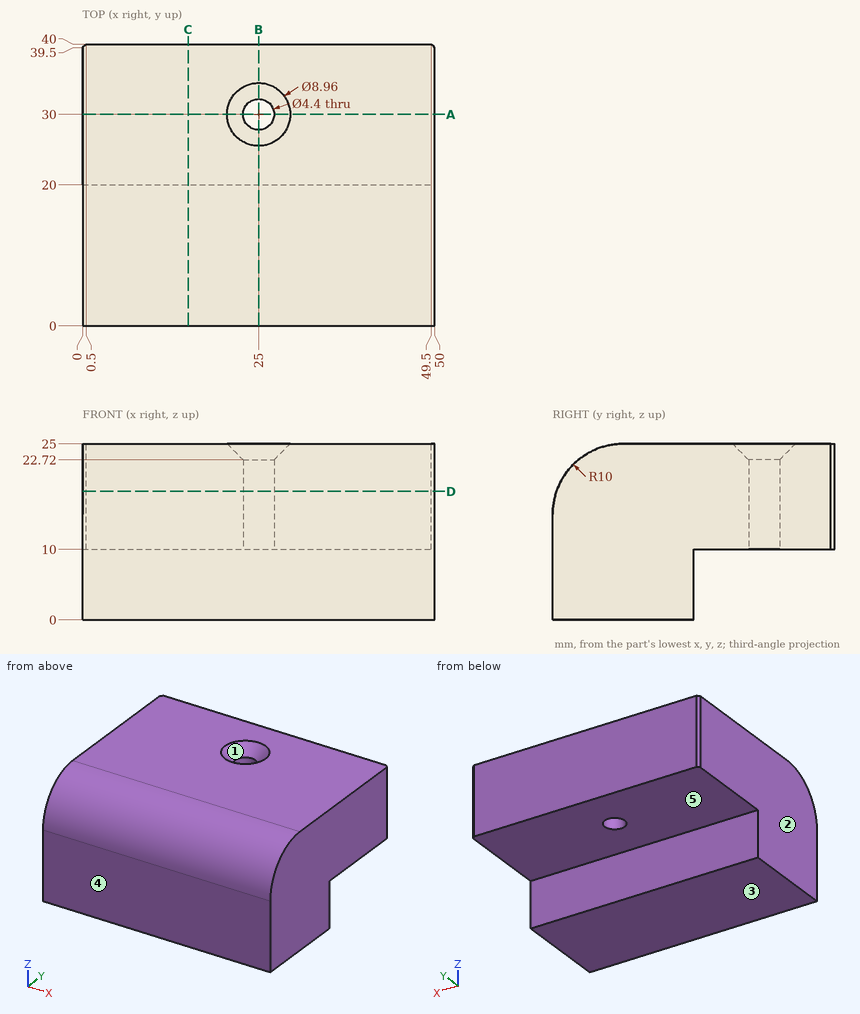
Study the drawing (mm; zero at the part's minimum x, y, z) and answer. A direction names the side the tool comes from. Coordinates: 2 decimals unless noted, no trailing zeros. Write each loop counter-clockwise with the first axis right and the second up, starting at its lowest first coordinate (ties: lowest second). Pieces come first, ordered by that corner, then holes. Notation, with made-up numbers: (-22.5, 50) - (-12.5, 50) arc R36 cw to (-12.5, 85) - close; hole circle Ø11 at (-6.75, 7). An arc over 180 degrees is marked (long way). Put each result on its own line as item: value.
1. Determine the mould class of the marked faces 1, 2 and 3 for opening direction X: pulls with the +X half, pulls with the -X half, needs draft (parallel to the pull), parting line crosses it, or undercut.
Answer sheet:
face 1: undercut
face 2: pulls with the -X half
face 3: needs draft
2. The part is cut by section C-C on x = 15. Give the vertices of the cut face in (y, z).
Answer sheet:
outline: (0, 0) - (20, 0) - (20, 10) - (40, 10) - (40, 25) - (10, 25) arc R10 ccw to (0, 15) - close
3. Find the intervals of material crossed by line 1 along Y through (x, z) = (25, 15); line 2 along X through (y, z) = (30, 16); line 3 along Z through (x, y) = (42, 29), in increasing order. Write a range as from..to.
Answer sheet:
line 1: y = 0..27.8, 32.2..40
line 2: x = 0..22.8, 27.2..50
line 3: z = 10..25
4. The part is cut by section B-B on x = 25. Give the vertices of the cut face in (y, z).
Answer sheet:
outline: (0, 0) - (20, 0) - (20, 10) - (27.8, 10) - (27.8, 22.72) - (25.52, 25) - (10, 25) arc R10 ccw to (0, 15) - close; (32.2, 10) - (40, 10) - (40, 25) - (34.48, 25) - (32.2, 22.72) - close
5. The part is cut by section A-A on y = 30. Give the vertices of the cut face in (x, z).
Answer sheet:
outline: (0, 10) - (22.8, 10) - (22.8, 22.72) - (20.52, 25) - (0, 25) - close; (27.2, 10) - (50, 10) - (50, 25) - (29.48, 25) - (27.2, 22.72) - close
6. A tool of negligible diameter and unlimited length cuts with its end or side. For the marked faces 4 and 5, from which of +Z, -Z, +X, -X, +Y, -Y can it reach the whole face along a straight path? Write none if from no direction.
Answer sheet:
face 4: +Z, -Z, +X, -X, -Y
face 5: -Z, +X, -X, +Y
7. The part is cut by section D-D on z = 18.25. Give the vertices of the cut face in (x, y), plus the area to 3 significant figures.
Answer sheet:
outline: (0, 0.54) - (50, 0.54) - (50, 39.5) - (49.5, 40) - (0.5, 40) - (0, 39.5) - close; hole circle Ø4.4 at (25, 30)
area: 1,960 mm^2
8. Flat-ended cylindrical pins translate along their axes: pin 1 Ø5 at (x, y) = (25, 30) entering from -Z; pin 2 Ø8 at (y, z) = (30.5, 4.5) entering from -X; pin 3 Ø1.5 at (x, z) = (33.5, 7) entering from +Y; pin 4 Ø5 at (x, y) = (14.5, 6.5) entering from +Z. Find the tip coordinate at first contact, or state that the pin passes through.
Answer sheet:
pin 1: stops at z = 10
pin 2: passes through
pin 3: stops at y = 20
pin 4: stops at z = 24.95
